```python
from build123d import *

# Parameters (mm, degrees)
EXTRUDE_1_DEPTH        = 26
EXTRUDE_2_DEPTH        = 19
FILLET_1_R             = 10
SKETCH_5_W             = 161
SKETCH_5_H             = 6
CUT_EXTRUDE_1_DEPTH    = 52
SKETCH_1_5_W           = 11
SKETCH_1_5_H           = 340
EXTRUDE_4_DEPTH        = 7
SKETCH_6_W             = 1.9
SKETCH_6_H             = 2
SKETCH_6_W_2           = 6.6
EXTRUDE_5_DEPTH        = 28
SKETCH_6_3_W           = 6.6
SKETCH_6_3_H           = 2
CUT_EXTRUDE_2_DEPTH    = 5
FILLET_2_R             = 20
SKETCH_6_4_W           = 15
SKETCH_6_4_H           = 10
SKETCH_6_4_H_2         = 9
EXTRUDE_6_DEPTH        = 30
SKETCH_6_5_W           = 15
SKETCH_6_5_H           = 9
EXTRUDE_7_DEPTH        = 28
EXTRUDE_8_DEPTH        = 15
FILLET_3_R             = 20
FILLET_3_OF_MIRROR_2_R = 20
FILLET_4_R             = 20
SKETCH_11_W            = 20
SKETCH_11_H            = 20
CUT_EXTRUDE_3_DEPTH    = 617
SKETCH_10_W            = 20
SKETCH_10_H            = 10
CUT_EXTRUDE_4_DEPTH    = 617
SKETCH_13_W            = 2
SKETCH_13_H            = 9
CUT_EXTRUDE_8_DEPTH    = 8.5


with BuildPart() as part:
    # 스케치1 → 보스-돌출1 (new body)
    with BuildSketch(Plane.XY):
        Polygon((-168, 0), (168, 0), (183, 0), (183, -340), (168, -340), (168, -20), (-168, -20), (-168, -340), (-183, -340), (-183, 0), align=None)
    extrude(amount=EXTRUDE_1_DEPTH)

    # 스케치1<4> → 보스-돌출2 (add)
    with BuildSketch(Plane.XY):
        Polygon((172, 0), (168, 0), (168, -20), (168, -340), (172, -340), align=None)
        Polygon((-168, -20), (-168, 0), (-172, 0), (-172, -340), (-168, -340), align=None)
    extrude(amount=-EXTRUDE_2_DEPTH)

    # 필렛1
    fillet_1_edges = [part.edges().sort_by_distance(p)[0] for p in [
        (170, 0, -19),
        (170, -340, -19),
        (-170, -340, -19),
        (-170, 0, -19),
    ]]
    fillet(fillet_1_edges, radius=FILLET_1_R)

    # 스케치5 → 컷-돌출1 (cut)
    with BuildSketch(Plane(origin=(0, 0, 0), x_dir=(1, 0, 0), z_dir=(0, 1, 0))):
        with Locations((-87.5, -3)):
            Rectangle(SKETCH_5_W, SKETCH_5_H)
        with Locations((87.5, -3)):
            Rectangle(SKETCH_5_W, SKETCH_5_H)
    extrude(amount=-CUT_EXTRUDE_1_DEPTH, mode=Mode.SUBTRACT)

    # 스케치1<5> → 보스-돌출4 (add)
    with BuildSketch(Plane.XY):
        with Locations((177.5, -170)):
            Rectangle(SKETCH_1_5_W, SKETCH_1_5_H)
        with Locations((-177.5, -170)):
            Rectangle(SKETCH_1_5_W, SKETCH_1_5_H)
    extrude(amount=-EXTRUDE_4_DEPTH)

    # 스케치6 → 보스-돌출5 (add)
    with BuildSketch(Plane.XZ.offset(340)):
        with Locations((-182.05, -6)):
            Rectangle(SKETCH_6_W, SKETCH_6_H)
        with Locations((-177.8, -6)):
            Rectangle(SKETCH_6_W_2, SKETCH_6_H)
        Polygon((-174.5, -7), (-172, -7), (-168, -7), (-168, -5), (-174.5, -5), align=None)
    extrude_5 = extrude(amount=EXTRUDE_5_DEPTH)

    # 스케치6<3> → 컷-돌출2 (cut)
    with BuildSketch(Plane.XZ.offset(340)):
        with Locations((-177.8, -6)):
            Rectangle(SKETCH_6_3_W, SKETCH_6_3_H)
    cut_extrude_2 = extrude(amount=CUT_EXTRUDE_2_DEPTH, mode=Mode.SUBTRACT)

    # 필렛2
    # the kernel refuses this fillet: 20 mm, written as the material it adds along each edge
    with BuildSketch(Plane(origin=(-172, -340, -7), x_dir=(0, -1, 0), z_dir=(1, 0, 0))) as fillet_2_piece_1:
        with BuildLine():
            CenterArc((14, 20), FILLET_2_R, 216.869897646, 53.130102354)
            Line((-2, 8), (-3.6, 6.8))
            ThreePointArc((-3.6, 6.8), (-2, 2), (-2, 0))
            Line((-2, 0), (0, -2))
            Line((0, -2), (14, -2))
            Line((14, -2), (14, 0))
        make_face()
    extrude(amount=4)

    # 스케치6<4> → 보스-돌출6 (add)
    with BuildSketch(Plane.XZ.offset(340)):
        with Locations((-175.5, 31)):
            Rectangle(SKETCH_6_4_W, SKETCH_6_4_H)
        with Locations((-175.5, 40.5)):
            Rectangle(SKETCH_6_4_W, SKETCH_6_4_H_2)
    extrude_6 = extrude(amount=-EXTRUDE_6_DEPTH)

    # 스케치6<5> → 보스-돌출7 (add)
    with BuildSketch(Plane.XZ.offset(340)):
        with Locations((-175.5, 40.5)):
            Rectangle(SKETCH_6_5_W, SKETCH_6_5_H)
    extrude_7 = extrude(amount=EXTRUDE_7_DEPTH)

    # 스케치9 → 보스-돌출8 (add)
    with BuildSketch(Plane.ZY.offset(183)):
        Polygon((26, -310), (45, -310), (26, -270), align=None)
    extrude_8 = extrude(amount=-EXTRUDE_8_DEPTH)

    # 필렛3
    fillet_3_edges = [part.edges().sort_by_distance(p)[0] for p in [
        (-175.5, -310, 45),
        (-175.5, -270, 26),
    ]]
    fillet(fillet_3_edges, radius=FILLET_3_R)

    # 대칭 복사2: 보스-돌출5, 컷-돌출2, 보스-돌출6, 보스-돌출7, 보스-돌출8 across plane
    add(extrude_5.mirror(Plane(origin=(0, 0, 0), x_dir=(0, 0, 1), z_dir=(1, 0, 0))))
    add(cut_extrude_2.mirror(Plane(origin=(0, 0, 0), x_dir=(0, 0, 1), z_dir=(1, 0, 0))), mode=Mode.SUBTRACT)
    add(extrude_6.mirror(Plane(origin=(0, 0, 0), x_dir=(0, 0, 1), z_dir=(1, 0, 0))))
    add(extrude_7.mirror(Plane(origin=(0, 0, 0), x_dir=(0, 0, 1), z_dir=(1, 0, 0))))
    add(extrude_8.mirror(Plane(origin=(0, 0, 0), x_dir=(0, 0, 1), z_dir=(1, 0, 0))))

    # 필렛3 of 대칭 복사2
    fillet_3_of_mirror_2_edges = [part.edges().sort_by_distance(p)[0] for p in [
        (175.5, -310, 45),
        (175.5, -270, 26),
    ]]
    fillet(fillet_3_of_mirror_2_edges, radius=FILLET_3_OF_MIRROR_2_R)

    # 필렛4
    # the kernel refuses this fillet: 20 mm, written as the material it adds along each edge
    with BuildSketch(Plane(origin=(172, -340, -7), x_dir=(0, 0.24253562503633938, -0.9701425001453302), z_dir=(-1, 0, 0))) as fillet_4_piece_1:
        with BuildLine():
            CenterArc((16.007351252, 18.432707503), FILLET_4_R, 194.036243468, 53.130102354)
            Line((-3.395498751, 13.581995002), (-5.335783751, 13.096923752))
            Line((-5.335783751, 13.096923752), (-1.940285, -0.48507125))
            Line((-1.940285, -0.48507125), (0.48507125, -1.940285))
            ThreePointArc((0.48507125, -1.940285), (2.42535625, -1.45521375), (7.470097251, -1.84327075))
            Line((7.470097251, -1.84327075), (8.246211251, 0))
        make_face()
    extrude(amount=4)

    # 스케치11 → 컷-돌출3 (cut)
    with BuildSketch(Plane.ZY.offset(-168)):
        with BuildLine():
            ThreePointArc((45, -314.508610159), (44.510394688, -310.110371974), (43.065550087, -305.927473868))
            Line((43.065550087, -305.927473868), (27.934449913, -274.072526132))
            ThreePointArc((27.934449913, -274.072526132), (26.489605312, -269.889628026), (26, -265.491389841))
            Line((26, -265.491389841), (26, -20))
            Line((26, -20), (6, -20))
            Line((6, -20), (6, 0))
            Line((6, 0), (-7, 0))
            Line((-7, 0), (-7, -354))
            Line((-7, -354), (-7, -368))
            Line((-7, -368), (-5, -368))
            Line((-5, -368), (-5, -340))
            Line((-5, -340), (36, -340))
            Line((36, -340), (36, -368))
            Line((36, -368), (45, -368))
            Line((45, -368), (45, -314.508610159))
        make_face()
        with Locations((16, -10)):
            Rectangle(SKETCH_11_W, SKETCH_11_H)
        with BuildLine():
            Line((-7, -354), (-7, 0))
            Line((-7, 0), (-9, 0))
            ThreePointArc((-9, 0), (-16.071067812, -2.928932188), (-19, -10))
            Line((-19, -10), (-19, -330))
            ThreePointArc((-19, -330), (-17.94427191, -334.472135955), (-15, -338))
            ThreePointArc((-15, -338), (-9.11145618, -345.05572809), (-7, -354))
        make_face()
    extrude(amount=CUT_EXTRUDE_3_DEPTH, mode=Mode.SUBTRACT)

    # 스케치10 → 컷-돌출4 (cut)
    with BuildSketch(Plane(origin=(183, 0, 0), x_dir=(0, 0, -1), z_dir=(1, 0, 0))):
        with Locations((-16, -15)):
            Rectangle(SKETCH_10_W, SKETCH_10_H)
    extrude(amount=-CUT_EXTRUDE_4_DEPTH, mode=Mode.SUBTRACT)

    # 스케치13 → 컷-돌출8 (cut)
    with BuildSketch(Plane(origin=(183, 0, 0), x_dir=(0, 0, -1), z_dir=(1, 0, 0))):
        with Locations((6, -344.5)):
            Rectangle(SKETCH_13_W, SKETCH_13_H)
    extrude(amount=-CUT_EXTRUDE_8_DEPTH, mode=Mode.SUBTRACT)


solid = part.part
```
The listing builds one solid part. Answer for the finished solid, in the listing's coordinates (mm). A direction names the side the tool comes from. Coordinates: 2 decimals unless noted, no trailing zeros. Loops run counter-clockwise (first coordinate to the right, second up) from the corner with the lowest first, then second, coordinate; pieces in that order, holes last. Notation, with made-up numbers: (-19, -32) -> (7, -32) arc R15 ccw to (7, -5) -> close; hole circle Ø7 at (-29.75, -22). An arc over 180 degrees is marked (long way). Return JSON: item names as keys, results as strings. Group by question number.
(1) A cutting plane is placed at B-B on z = 18.5. Write down the section's boundary in (x, y), and give its area (3 significant figures).
(2) A cutting plane is placed at D-D on y = -300.5. Write down the section's boundary in (x, z).
(3) Determine the mould class of faces 1 (the flat face through (176, -20, 16)), 2 (the flat face through (176, -141, 26)), 3 (the flat face through (176, -354, 36)) for opening direction Z: released by +Z, released by -Z, zero draft, split by the parting line, or undercut.
(4) A cutting plane is placed at C-C on y = -164. Write down the section's boundary in (x, z).
(5) Given pin 1 Ø7.5 at (x, z) = (174, 24.5) entering from -Y; pin 2 Ø3 at (x, y) = (172.5, -13.5) entering from +Z; pin 3 Ø1 at (y, z) = (-344, -6) entering from +X, each flat-ended and moving along its own axis, determine where each tip first touches the part or whether it passes through.
(6) Find the intervals of material crossed by probe 1 along Y at (x, z) = (182.25, 21.5); probe 2 along Z at (x, y) = (173, -129); probe 3 along Y at (x, z) = (180.5, -1), in increasing order. Write a range as from..to.
(7) Which of the six approach directions +Z, -Z, +X, -X, +Y, -Y give full straight-line access (tool end or side, diameter ignored) to faces 4 (the cylindrical face through (170.028, -345.172, -9.054)), 5 (the flat face through (176, -15, 6)), 6 (the flat face through (176, -5, 26)), 7 (the cylindrical face through (169.97, -2.85, -15.99)), 8 (the flat face through (175, -357, -5))?
(8) A cutting plane is placed at A-A on x = 178.5. Write down the section's boundary in (y, z), and give its area (3 significant figures).
The answers:
{
 "1": {"outline": "(168, -340) -> (183, -340) -> (183, -20) -> (168, -20) -> close; (168, -10) -> (183, -10) -> (183, 0) -> (168, 0) -> close", "area": "4,950 mm^2"},
 "2": {"outline": "(168, -19) -> (172, -19) -> (172, -7) -> (183, -7) -> (183, 40.49) -> (168, 40.49) -> close"},
 "3": {"face 1": "zero draft", "face 2": "released by +Z", "face 3": "undercut"},
 "4": {"outline": "(168, -19) -> (172, -19) -> (172, -7) -> (183, -7) -> (183, 26) -> (168, 26) -> close"},
 "5": {"pin 1": "stops at y = -340", "pin 2": "stops at z = 6", "pin 3": "stops at x = 174.5"},
 "6": {"probe 1": "y = -340..-20, -10..0", "probe 2": "z = -7..26", "probe 3": "y = -340..0"},
 "7": {"face 4": "-Z, +X, -X, -Y", "face 5": "+Z, +X, -X", "face 6": "+Z, +X, -X, +Y", "face 7": "-Z, +X, -X, +Y", "face 8": "+X, -X, -Y"},
 "8": {"outline": "(-368, -7) -> (-349, -7) -> (-349, -5) -> (-368, -5) -> close; (-368, 36) -> (-340, 36) -> (-340, -7) -> (0, -7) -> (0, 26) -> (-10, 26) -> (-10, 6) -> (-20, 6) -> (-20, 26) -> (-265.49, 26) arc R20 cw to (-274.07, 27.93) -> (-305.93, 43.07) arc R20 ccw to (-314.51, 45) -> (-368, 45) -> close", "area": "12,300 mm^2"}
}
